Design review of the part built by this model. Coordinates are the model's own, in mm. A direction names the side the tool comes from. Give positions to 0.01 mm unless a question says otherwise; leave off trailing zeros. Order: outer loops, then holes, each group sorted by start corner. A loop starts at its lowest first (then second) coordinate and runs counter-clockwise, first axis right, second up.
```python
from build123d import *

# Parameters (mm, degrees)
SKETCH1_R           = 10
BOSS_EXTRUDE1_DEPTH = 100
SKETCH2_R           = 20
BOSS_EXTRUDE3_DEPTH = 700
SKETCH4_OUTSIDE_W   = 324.884
SKETCH4_OUTSIDE_H   = 324.884
SKETCH4_OUTSIDE_R   = 10.5
CUT_EXTRUDE2_DEPTH  = 700
CUT_EXTRUDE2_DRAFT  = -5


with BuildPart() as part:
    # Sketch1 → Boss-Extrude1 (new body)
    with BuildSketch(Plane(origin=(0, 0, 0), x_dir=(0, 0, -1), z_dir=(1, 0, 0))):
        Circle(SKETCH1_R)
    extrude(amount=BOSS_EXTRUDE1_DEPTH)

    # Sketch2 → Boss-Extrude3 (add)
    with BuildSketch(Plane(origin=(100, 0, 0), x_dir=(0, 0, -1), z_dir=(1, 0, 0))):
        Circle(SKETCH2_R)
    extrude(amount=BOSS_EXTRUDE3_DEPTH)


with BuildPart() as cut_extrude2_tool:
    # Sketch4 outside → Cut-Extrude2 (with draft: the straight prism first)
    with BuildSketch(Plane.ZY.offset(-100)):
        Rectangle(SKETCH4_OUTSIDE_W, SKETCH4_OUTSIDE_H)
        Circle(SKETCH4_OUTSIDE_R, mode=Mode.SUBTRACT)
    extrude(amount=-CUT_EXTRUDE2_DEPTH)
    # Cut-Extrude2: the draft: its side faces are tilted about the plane it starts from
    cut_extrude2_sides = [cut_extrude2_tool.faces().sort_by_distance(p)[0] for p in [
        (450, -162.442, 0),
        (450, 0, 162.442),
        (450, 162.442, 0),
        (450, 0, -162.442),
        (450, 0, -10.5),
    ]]
    draft(cut_extrude2_sides, Plane.ZY.offset(-100), CUT_EXTRUDE2_DRAFT)


with BuildPart() as part_1:
    add(part.part)

    # Cut-Extrude2: cut by cut_extrude2_tool
    add(cut_extrude2_tool.part, mode=Mode.SUBTRACT)


solid = part_1.part
```
1. Take a section at A-A (z = 0). State the section outline as (x, y) points, then the cut area to 3 significant figures.
Recorded:
outline: (0, -10) - (100, -10) - (100, -10.5) - (208.59, -20) - (800, -20) - (800, 20) - (208.59, 20) - (100, 10.5) - (100, 10) - (0, 10) - close
area: 29,000 mm2
2. For line 1 along Z through (x, y) = (113, 6); line 2 along Z through (x, y) = (668.5, -1), list the stretches that pass through material, from the lowest coordinate up.
Recorded:
line 1: z = -9.97 to 9.97
line 2: z = -19.97 to 19.97
3. For pin 1 (4 mm diameter, centred on x = 472, z = 12, fed in from -Y); pin 2 (5 mm diameter, centred on x = 162, y = 9.5, fed in from -Z); pin 3 (2 mm diameter, centred on x = 92, y = -3, fed in from -Z), all flat-tipped, find the tip position at first contact; note any pin that passes through.
Recorded:
pin 1: stops at y = -17.32
pin 2: stops at z = -14.33
pin 3: stops at z = -9.8
4. Take a section at C-C (x = 417.5). State the section outline as (y, z) points.
Recorded:
outline: circle Ø40 at (0, 0)
5. Machinability: for faces 1 (the face through (500.153, -19.524, 4.336)), 2 (the face through (100, -9, -5)), which of the approach directions +Z, -Z, +X, -X, +Y, -Y give a long, thin tool a straight path to every point of the face, cutting with its end or side? Answer none if there is none.
Recorded:
face 1: +X, -X
face 2: -X
6. Take a section at D-D (x = 108). State the section outline as (y, z) points.
Recorded:
outline: circle Ø22.4 at (0, 0)
